Verification items for the finished model (mm, model axes). Round coordinates to 2 decimals unless told otherwise and drop trailing zeros. Order: outer loops, then holes, each group sorted by start corner. A loop starts at its lowest first (then second) coordinate and runs counter-clockwise, first axis right, second up. Notation, with made-up numbers: M 81.25,21 L 140.25,21 A18 cw 140.25,55 Z; hole C 12.5,88 d1. An arc over 180 degrees is marked long. Use CSV: the item, a comma, the result in double quotes. Start each with the question number.
Q1. Sectioned sample at B-B (z = 0.8). State how many separate pieces and enclosed holes the cut face has, and give its area (3 significant figures).
Q2. Scan lines: line 1 (X direction, y = -56.5, z = 0.7); line 2 (Y direction, x = 12, z = 2.2); line 3 (X direction, y = 53.5, z = 0.1). Record each from-to range of solid material in increasing order.
Q3. Sectioned sample at A-A (y = 8). Enter the section's corners in (x, z).
Q4. Gauge pin test, flat ends, axial feed: pin 1 Ø0.9 at (y, z) = (40, 2) entering from -X; pin 2 Ø8 at (x, y) = (14.5, 8) entering from -Z; pin 3 Ø1.5 at (y, z) = (-52.5, 1.5) entering from +X. Record the tip position at first contact, or that the pin passes through.
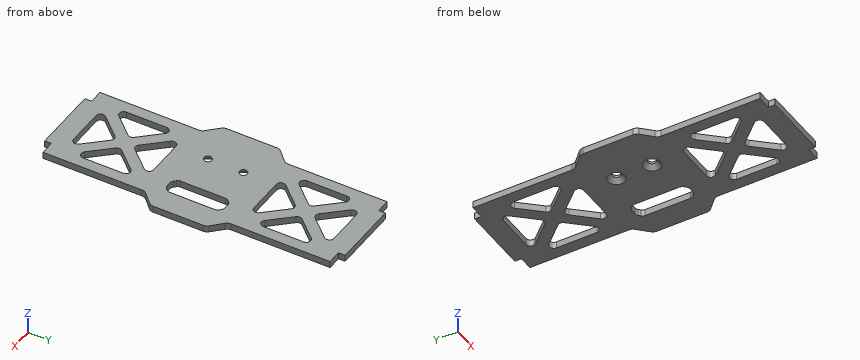
```python
from build123d import *

# Parameters (mm, degrees)
SKETCH_1_W          = 55
SKETCH_1_H          = 129
SKETCH_1_W_2        = 30
SKETCH_1_H_2        = 6
EXTRUDE_1_DEPTH     = 3
SKETCH_2_R          = 1.75
CUT_EXTRUDE_1_DEPTH = 10
CUT_EXTRUDE_2_DEPTH = 10
FILLET_1_R          = 3
CHAMFER_1_SIZE      = 2
CUT_EXTRUDE_3_DEPTH = 10
FILLET_2_R          = 2


with BuildPart() as part:
    # Эскиз1 → Бобышка-Вытянуть1 (new body)
    with BuildSketch(Plane.XY):
        Rectangle(SKETCH_1_W, SKETCH_1_H)
        with Locations((0, 64.5)):
            Rectangle(SKETCH_1_W_2, SKETCH_1_H_2)
        with Locations((0, -64.5)):
            Rectangle(SKETCH_1_W_2, SKETCH_1_H_2)
    extrude(amount=EXTRUDE_1_DEPTH)

    # Эскиз2 → Вырез-Вытянуть1 (cut)
    with BuildSketch(Plane.XY.offset(3)):
        with Locations((-8, 8)):
            Circle(SKETCH_2_R)
        with Locations((-8, -8)):
            Circle(SKETCH_2_R)
    extrude(amount=-CUT_EXTRUDE_1_DEPTH, mode=Mode.SUBTRACT)

    # Эскиз3 → Вырез-Вытянуть2 (cut)
    with BuildSketch(Plane.XY.offset(3)):
        Polygon((-21.25, 64.5), (-21.25, 18.75), (-27.5, 12.5), (-35.562933311, 12.5), (-37.53189801, 71.38735117), align=None)
        Polygon((35.562933311, 12.5), (27.5, 12.5), (21.25, 18.75), (21.25, 64.5), (37.53189801, 71.38735117), align=None)
        Polygon((21.25, -64.5), (21.25, -18.75), (27.5, -12.5), (35.562933311, -12.5), (37.53189801, -71.38735117), align=None)
        Polygon((-35.562933311, -12.5), (-27.5, -12.5), (-21.25, -18.75), (-21.25, -64.5), (-37.53189801, -71.38735117), align=None)
    extrude(amount=-CUT_EXTRUDE_2_DEPTH, mode=Mode.SUBTRACT)

    # Скругление1
    fillet_1_edges = [part.edges().sort_by_distance(p)[0] for p in [
        (-21.25, 18.75, 1.5),
        (-27.5, 12.5, 1.5),
        (-27.5, -12.5, 1.5),
        (-21.25, -18.75, 1.5),
        (21.25, -18.75, 1.5),
        (27.5, -12.5, 1.5),
        (27.5, 12.5, 1.5),
        (21.25, 18.75, 1.5),
    ]]
    fillet(fillet_1_edges, radius=FILLET_1_R)

    # Фаска1
    chamfer_1_edges = [part.edges().sort_by_distance(p)[0] for p in [
        (-9.75, 8, 0),
        (-9.75, -8, 0),
    ]]
    chamfer(chamfer_1_edges, length=CHAMFER_1_SIZE)

    # Эскиз4 → Вырез-Вытянуть3 (cut)
    with BuildSketch(Plane.XY.offset(3)):
        Polygon((12.881944444, 22.5), (0, 36.769230769), (-12.881944444, 22.5), align=None)
        Polygon((-3.368055556, 40.5), (-16.25, 54.769230769), (-16.25, 26.230769231), align=None)
        Polygon((12.881944444, 58.5), (-12.881944444, 58.5), (0, 44.230769231), align=None)
        Polygon((16.25, 54.769230769), (3.368055556, 40.5), (16.25, 26.230769231), align=None)
        Polygon((15, -13), (11, -13), (9, -11), (9, 11), (11, 13), (15, 13), (17, 11), (17, -11), align=None)
        Polygon((-12.881944444, -22.5), (0, -36.769230769), (12.881944444, -22.5), align=None)
        Polygon((16.25, -26.230769231), (3.368055556, -40.5), (16.25, -54.769230769), align=None)
        Polygon((12.881944444, -58.5), (0, -44.230769231), (-12.881944444, -58.5), align=None)
        Polygon((-3.368055556, -40.5), (-16.25, -26.230769231), (-16.25, -54.769230769), align=None)
    extrude(amount=-CUT_EXTRUDE_3_DEPTH, mode=Mode.SUBTRACT)

    # Скругление2
    fillet_2_edges = [part.edges().sort_by_distance(p)[0] for p in [
        (16.25, -54.769230769, 1.5),
        (3.368055556, -40.5, 1.5),
        (16.25, -26.230769231, 1.5),
        (-12.881944444, -22.5, 1.5),
        (12.881944444, -22.5, 1.5),
        (0, -36.769230769, 1.5),
        (-16.25, -54.769230769, 1.5),
        (-16.25, -26.230769231, 1.5),
        (-3.368055556, -40.5, 1.5),
        (-12.881944444, -58.5, 1.5),
        (0, -44.230769231, 1.5),
        (12.881944444, -58.5, 1.5),
        (0, 44.230769231, 1.5),
        (-12.881944444, 58.5, 1.5),
        (12.881944444, 58.5, 1.5),
        (-16.25, 26.230769231, 1.5),
        (-16.25, 54.769230769, 1.5),
        (-3.368055556, 40.5, 1.5),
        (3.368055556, 40.5, 1.5),
        (16.25, 54.769230769, 1.5),
        (16.25, 26.230769231, 1.5),
        (15, -13, 1.5),
        (11, -13, 1.5),
        (9, -11, 1.5),
        (9, 11, 1.5),
        (11, 13, 1.5),
        (15, 13, 1.5),
        (17, 11, 1.5),
        (17, -11, 1.5),
        (-12.881944444, 22.5, 1.5),
        (0, 36.769230769, 1.5),
        (12.881944444, 22.5, 1.5),
    ]]
    fillet(fillet_2_edges, radius=FILLET_2_R)


solid = part.part
```
Verdict:
1,separate pieces,"1"
1,enclosed holes,"11"
1,area,"4,420 mm²"
2,line 1,"x = -21.25 to -10.38, 10.38 to 21.25"
2,line 2,"y = -67.5 to -50.06, -30.94 to -13, 13 to 30.94, 50.06 to 67.5"
2,line 3,"x = -21.25 to -8.37, 8.37 to 21.25"
3,outline,"M -27.5,0 L -11.75,0 L -9.75,2 L -9.75,3 L -27.5,3 Z; M -6.25,2 L -4.25,0 L 9,0 L 9,3 L -6.25,3 Z; M 17,0 L 27.5,0 L 27.5,3 L 17,3 Z"
4,pin 1,"stops at x = -21.25"
4,pin 2,"stops at z = 0"
4,pin 3,"stops at x = 21.25"
